The model under review builds one solid part; all positions refer to its coordinate system, in mm. Give positions to 0.01 mm unless a question says otherwise; leave off trailing zeros. Order: outer loops, then holes, each group sorted by start corner. A loop starts at its lowest first (then second) coordinate and runs counter-clockwise, first axis right, second up.
```python
from build123d import *
from OCP.BRepFilletAPI import BRepFilletAPI_MakeChamfer

# Parameters (mm, degrees)
BOSS_EXTRUDE1_DEPTH = 6.35
CHAMFER1_SIZE       = 1.5875
CHAMFER1_SIZE2      = 2.749630657
CHAMFER2_SIZE       = 2.7432
CHAMFER2_SIZE2      = 1.583787258
FILLET1_R           = 10


with BuildPart() as part:
    # Sketch1 → Boss-Extrude1 (new body)
    with BuildSketch(Plane.XY):
        with BuildLine():
            Line((-19.05, 0), (-19.05, 31.75))
            Line((-19.05, 31.75), (31.75, 31.75))
            Line((31.75, 31.75), (31.75, -19.05))
            Line((31.75, -19.05), (0, -19.05))
            ThreePointArc((0, -19.05), (-13.470384182, -13.470384182), (-19.05, 0))
        make_face()
    extrude(amount=BOSS_EXTRUDE1_DEPTH)

    # Chamfer1: one chamfer whose edges measure the first distance from different faces: ONE call of the kernel's chamfer builder (chamfer() names one face for all edges)
    chamfer1_edges_1 = [part.edges().sort_by_distance(p)[0] for p in [
        (-19.05, 15.875, 6.35),
    ]]
    chamfer1_side_1 = [part.faces().sort_by_distance(p)[0] for p in [
        (-19.05, 15.875, 3.175),
    ]]
    chamfer1_edges_2 = [part.edges().sort_by_distance(p)[0] for p in [
        (-13.470384182, -13.470384182, 6.35),
    ]]
    chamfer1_side_2 = [part.faces().sort_by_distance(p)[0] for p in [
        (-13.470384182, -13.470384182, 3.175),
    ]]
    chamfer1_edges_3 = [part.edges().sort_by_distance(p)[0] for p in [
        (15.875, -19.05, 6.35),
    ]]
    chamfer1_side_3 = [part.faces().sort_by_distance(p)[0] for p in [
        (15.875, -19.05, 3.175),
    ]]
    chamfer1 = BRepFilletAPI_MakeChamfer(part.part.solid().wrapped)
    for e in chamfer1_edges_1:
        chamfer1.Add(CHAMFER1_SIZE, CHAMFER1_SIZE2, e.wrapped, chamfer1_side_1[0].wrapped)  # the first distance lies on this face
    for e in chamfer1_edges_2:
        chamfer1.Add(CHAMFER1_SIZE, CHAMFER1_SIZE2, e.wrapped, chamfer1_side_2[0].wrapped)  # the first distance lies on this face
    for e in chamfer1_edges_3:
        chamfer1.Add(CHAMFER1_SIZE, CHAMFER1_SIZE2, e.wrapped, chamfer1_side_3[0].wrapped)  # the first distance lies on this face
    add(Compound.cast(chamfer1.Shape()), mode=Mode.REPLACE)

    # Chamfer2
    chamfer2_edges = [part.edges().sort_by_distance(p)[0] for p in [
        (-19.05, 15.875, 0),
        (15.875, -19.05, 0),
        (-13.470384182, -13.470384182, 0),
    ]]
    chamfer2_side = [part.faces().sort_by_distance(p)[0] for p in [
        (7.007973691, 7.007973691, 0),
    ]]
    chamfer(chamfer2_edges, length=CHAMFER2_SIZE, length2=CHAMFER2_SIZE2, reference=chamfer2_side[0])

    # Fillet1
    fillet1_edges = [part.edges().sort_by_distance(p)[0] for p in [
        (31.75, -19.05, 3.173143629),
        (-19.05, 31.75, 3.173143629),
    ]]
    fillet(fillet1_edges, radius=FILLET1_R)


solid = part.part
```
Item 1: Take a section at C-C (x = 27.5). Give the boundary of the cut face in (y, z), and give its area (3 significant figures).
Values found:
outline: (-17.23, 0.53) - (-16.31, 0) - (31.75, 0) - (31.75, 6.35) - (-16.3, 6.35) - (-17.23, 5.81) - close
area: 311 mm2
Item 2: Take a section at B-B (y = 26). Give the boundary of the cut face in (x, z), and give its area (3 significant figures).
Values found:
outline: (-18.1, 1.04) - (-16.31, 0) - (31.75, 0) - (31.75, 6.35) - (-16.3, 6.35) - (-18.1, 5.31) - close
area: 315 mm2
Item 3: Clearance check with flat-ended pins moving along their axes: pin 1 Ø1.5 at (y, z) = (-11, 1) entering from -X; pin 2 Ø1.5 at (y, z) = (-12.5, 4.5) entering from -X. State where each tip first meets the part, or that it passes through.
Values found:
pin 1: stops at x = -15.88
pin 2: stops at x = -14.99
Item 4: For line 1 (Y direction, x = 4, z = 6); line 2 (Y direction, x = 25, z = 2.75); line 3 (X direction, y = -7, z = 0.5), list the stretches that pass through material, from the lowest coordinate up.
Values found:
line 1: y = -16.91 to 31.75
line 2: y = -18.51 to 31.75
line 3: x = -15.68 to 31.75
Item 5: Take a section at A-A (z = 2.5). Give the boundary of the cut face in (x, y).
Values found:
outline: (-19.05, 0) arc R19.05 ccw to (0, -19.05) - (21.75, -19.05) arc R10 ccw to (31.75, -9.05) - (31.75, 31.75) - (-9.05, 31.75) arc R10 ccw to (-19.05, 21.75) - close
